```python
from build123d import *

# Parameters (mm, degrees)
F0_R     = 1.5
F1_DEPTH = 2.4
F2_SIZE  = 0.25
F3_SIZE  = 0.25


with BuildPart() as f1:
    # F0 (on Top) → F1 (new body)
    with BuildSketch(Plane.XY):
        Polygon((0.298511, -2.985112), (2.734438, -1.234037), (2.435927, 1.751074), (-0.298511, 2.985112), (-2.734438, 1.234037), (-2.435927, -1.751074), align=None)
        Circle(F0_R, mode=Mode.SUBTRACT)
    extrude(amount=F1_DEPTH)

    # F2
    f2_edges = [f1.edges().sort_by_distance(p)[0] for p in [
        (-1.068708, -2.368093, 0),
        (1.516475, -2.109574, 0),
        (2.585182, 0.258518, 0),
        (1.068708, 2.368093, 0),
        (-1.516475, 2.109574, 0),
        (-2.585182, -0.258518, 0),
        (-1.5, 0, 0),
    ]]
    chamfer(f2_edges, length=F2_SIZE)

    # F3
    f3_edges = [f1.edges().sort_by_distance(p)[0] for p in [
        (-1.068708, -2.368093, 2.4),
        (1.516475, -2.109574, 2.4),
        (2.585182, 0.258518, 2.4),
        (1.068708, 2.368093, 2.4),
        (-1.516475, 2.109574, 2.4),
        (-2.585182, -0.258518, 2.4),
        (-1.5, 0, 2.4),
    ]]
    chamfer(f3_edges, length=F3_SIZE)


solid = f1.part
```
Verification items for the finished model (mm, model axes). Give positions to 0.01 mm unless a question says otherwise; leave off trailing zeros. Loops run counter-clockwise (first coordinate to the right, second up) from the corner with the lowest first, then second, coordinate; pieces in that order, holes last. Notation, with made-up numbers: M 58.25,7 L 62.25,7 A12 cw 62.25,17 Z; hole C 20.5,13 d7. An arc over 180 degrees is marked long. Return JSON: item names as keys, results as strings.
1) Material ranges on L1, parallel to Y at x = 0, z = 1.8; L2, parallel to Y at x = 1.3, z = 1.15; L3, parallel to X at y = 0.55, z = 0.6, recorded low to high. Write a range as [from, to].
Findings:
{"L1": "y = [-2.85, -1.5], [1.5, 2.85]", "L2": "y = [-2.27, -0.75], [0.75, 2.26]", "L3": "x = [-2.67, -1.4], [1.4, 2.56]"}
2) Section check B-B, the plane y = 0. Enter the section's corners in (x, z).
Findings:
{"outline": "M -2.61,0.25 L -2.36,0 L -1.75,0 L -1.5,0.25 L -1.5,2.15 L -1.75,2.4 L -2.36,2.4 L -2.61,2.15 Z; M 1.5,0.25 L 1.75,0 L 2.36,0 L 2.61,0.25 L 2.61,2.15 L 2.36,2.4 L 1.75,2.4 L 1.5,2.15 Z"}
3) Gauge pin test, flat end, axial feed: P1, Ø2.5, axis at x = 0, y = 0, coming from the -Z side. Record the tip position at first contact, or that the pin passes through.
Findings:
{"P1": "passes through"}
4) Section check C-C, the plane x = 0. Enter the section's corners in (y, z), and give its area (3 significant figures).
Findings:
{"outline": "M -2.85,0.25 L -2.58,0 L -1.75,0 L -1.5,0.25 L -1.5,2.15 L -1.75,2.4 L -2.58,2.4 L -2.85,2.15 Z; M 1.5,0.25 L 1.75,0 L 2.58,0 L 2.85,0.25 L 2.85,2.15 L 2.58,2.4 L 1.75,2.4 L 1.5,2.15 Z", "area": "6.22 mm2"}
5) Section check D-D, the plane y = 2.2. Enter the section's corners in (x, z).
Findings:
{"outline": "M -1.39,0.25 L -0.96,0 L 0.83,0 L 1.44,0.25 L 1.44,2.15 L 0.83,2.4 L -0.96,2.4 L -1.39,2.15 Z"}
6) Section check A-A, the plane z = 1.65. Enter the section's corners in (x, y).
Findings:
{"outline": "M -2.73,1.23 L -2.44,-1.75 L 0.3,-2.99 L 2.73,-1.23 L 2.44,1.75 L -0.3,2.99 Z; hole C 0,0 d3"}
